```python
from build123d import *

# Parameters (mm, degrees)
ESQUISSE1_R             = 1.6
EXTRUSION1_DEPTH        = 1
ESQUISSE2_W             = 59.55
ESQUISSE2_H             = 1
EXTRUSION2_DEPTH        = 7
ESQUISSE3_W             = 92.55
ESQUISSE3_H             = 1
EXTRUSION3_DEPTH        = 7.5
ESQUISSE4_W             = 92.55
ESQUISSE4_H             = 1
EXTRUSION4_DEPTH        = 8
CONG_1_R                = 1
CONG_2_R                = 2
CONG_3_R                = 1
CONG_4_R                = 2
ESQUISSE5_W             = 1.5
ESQUISSE5_H             = 17
ENL_V_MAT_EXTRU_1_DEPTH = 10
CONG_5_R                = 0.75
CONG_6_R                = 0.74
CONG_7_R                = 0.74
CONG_8_R                = 0.75


with BuildPart() as part:
    # Esquisse1 → Extrusion1 (new body)
    with BuildSketch(Plane.XY):
        Polygon((-46.275, -25.41), (-25.275, -25.41), (-25.275, -39.22), (34.275, -39.22), (34.275, -25.41), (46.275, -25.41), (46.275, -49.22), (-46.275, -49.22), align=None)
        with Locations((37.275, -29.41)):
            Circle(ESQUISSE1_R, mode=Mode.SUBTRACT)
        with Locations((-37.275, -29.41)):
            Circle(ESQUISSE1_R, mode=Mode.SUBTRACT)
    extrude(amount=EXTRUSION1_DEPTH)

    # Esquisse2 → Extrusion2 (add)
    with BuildSketch(Plane.XY.offset(1)):
        with Locations((4.5, -39.72)):
            Rectangle(ESQUISSE2_W, ESQUISSE2_H)
    extrude(amount=-EXTRUSION2_DEPTH)

    # Esquisse3 → Extrusion3 (add)
    with BuildSketch(Plane.XY.offset(1)):
        with Locations((0, -49.72)):
            Rectangle(ESQUISSE3_W, ESQUISSE3_H)
    extrude(amount=-EXTRUSION3_DEPTH)

    # Esquisse4 → Extrusion4 (add)
    with BuildSketch(Plane.XZ.offset(50.22)):
        with Locations((0, -6)):
            Rectangle(ESQUISSE4_W, ESQUISSE4_H)
    extrude(amount=EXTRUSION4_DEPTH)

    # Congé1
    cong_1_edges = [part.edges().sort_by_distance(p)[0] for p in [
        (0, -50.22, -5.5),
        (0, -49.22, 0),
    ]]
    fillet(cong_1_edges, radius=CONG_1_R)

    # Congé2
    cong_2_edges = [part.edges().sort_by_distance(p)[0] for p in [
        (0, -49.22, -6.5),
        (0, -50.22, 1),
    ]]
    fillet(cong_2_edges, radius=CONG_2_R)

    # Congé3
    cong_3_edges = [part.edges().sort_by_distance(p)[0] for p in [
        (4.5, -40.22, 0),
    ]]
    fillet(cong_3_edges, radius=CONG_3_R)

    # Congé4
    # the kernel refuses this fillet: 2 mm, written as the material it takes off along each edge
    with BuildSketch(Plane(origin=(-25.275, -39.22, 1), x_dir=(0, -1, 0), z_dir=(1, 0, 0))) as cong_4_piece_1:
        with BuildLine():
            CenterArc((CONG_4_R, CONG_4_R), CONG_4_R, 180, 90)
            Line((0, CONG_4_R), (0, 0))
            Line((0, 0), (CONG_4_R, 0))
        make_face()
    extrude(amount=59.55, mode=Mode.SUBTRACT)

    # Esquisse5 → Enlèv. mat.-Extru.1 (cut)
    with BuildSketch(Plane.XY.offset(1)):
        with Locations((-24.525, -33.91)):
            Rectangle(ESQUISSE5_W, ESQUISSE5_H)
        with Locations((33.525, -33.91)):
            Rectangle(ESQUISSE5_W, ESQUISSE5_H)
    extrude(amount=-ENL_V_MAT_EXTRU_1_DEPTH, mode=Mode.SUBTRACT)

    # Congé5
    cong_5_edges = [part.edges().sort_by_distance(p)[0] for p in [
        (-25.275, -42.41, 0.5),
    ]]
    fillet(cong_5_edges, radius=CONG_5_R)

    # Congé6
    cong_6_edges = [part.edges().sort_by_distance(p)[0] for p in [
        (-23.775, -42.41, 0.5),
    ]]
    fillet(cong_6_edges, radius=CONG_6_R)

    # Congé7
    cong_7_edges = [part.edges().sort_by_distance(p)[0] for p in [
        (32.775, -42.41, 0.5),
    ]]
    fillet(cong_7_edges, radius=CONG_7_R)

    # Congé8
    cong_8_edges = [part.edges().sort_by_distance(p)[0] for p in [
        (34.275, -42.41, 0.5),
    ]]
    fillet(cong_8_edges, radius=CONG_8_R)


solid = part.part
```
For this review, take the finished solid that the model builds, in its own axes (mm). A direction names the side the tool comes from. Round coordinates to 2 decimals unless told otherwise and drop trailing zeros. Loops run counter-clockwise (first coordinate to the right, second up) from the corner with the lowest first, then second, coordinate; pieces in that order, holes last.
Q1. Add section D-D on y = -47. Write out the cut boundary in (x, z) (3 decimals).
Result sheet:
outline: (-46.275, 0) - (46.275, 0) - (46.275, 1) - (-46.275, 1) - close
Q2. Mouldability with a two-part tool opening along Y and no side actions: class faces 5 (the face through (1, -42, 0)), 6 (the face through (-23.775, -40, -2)), 7 (the face through (4.1, -39.79, 0.4)) as +Y half, -Y half, draft (parallel to the pull), parting line (faces both ways), or undercut.
Result sheet:
face 5: undercut
face 6: draft
face 7: +Y half
Q3. Machinability: for faces 1 (the face through (-1, -55, -5.5)), 2 (the face through (0.65, -49.82, -5.93)), 3 (the face through (-1, -42, 1)), 4 (the face through (32.775, -40, -2)), which of the approach directions +Z, -Z, +X, -X, +Y, -Y give a long, thin tool a straight path to every point of the face, cutting with its end or side? Answer none if there is none.
Result sheet:
face 1: +Z, +X, -X, -Y
face 2: -Z, +X, -X
face 3: +Z, +X, -X, +Y, -Y
face 4: +Z, -Z, +Y
Q4. To check wall thickness, follow line 1 along X through (y, z) = (-35, 0.5) (3 decimals); line 2 along Y through (x, z) = (-16.5, -4.5); line 3 along Z through (x, y) = (-9, -42). State the ranges of each line that lie inside material, in increasing order.
Result sheet:
line 1: x = -46.275 to -25.275, 34.275 to 46.275
line 2: y = -50.22 to -49.22, -40.22 to -39.22
line 3: z = 0 to 1
Q5. Add section B-B on y = -29.41. Write out the cut boundary in (x, z) (3 decimals), plus the area to 3 significant figures.
Result sheet:
outline: (-46.275, 0) - (-38.875, 0) - (-38.875, 1) - (-46.275, 1) - close; (-35.675, 0) - (-25.275, 0) - (-25.275, 1) - (-35.675, 1) - close; (34.275, 0) - (35.675, 0) - (35.675, 1) - (34.275, 1) - close; (38.875, 0) - (46.275, 0) - (46.275, 1) - (38.875, 1) - close
area: 26.6 mm2
Q6. Insertion check: pin 1 Ø7 at (x, y) = (12.5, -38.5) entering from -Z; pin 2 Ø1.5 at (x, z) = (-1.5, -2.5) entering from -Y; pin 3 Ø4 at (x, z) = (25.5, -5) entering from +Y; pin 4 Ø5 at (x, y) = (34, -37) entering from +Z. Each pin has a flat end and moves straight along its axis. Give the tip position at first contact, or say it passes through.
Result sheet:
pin 1: stops at z = -6
pin 2: stops at y = -50.22
pin 3: stops at y = -39.22
pin 4: stops at z = 1
Q7. Add section A-A on y = -34. Write out the cut boundary in (x, z) (3 decimals).
Result sheet:
outline: (-46.275, 0) - (-25.275, 0) - (-25.275, 1) - (-46.275, 1) - close; (34.275, 0) - (46.275, 0) - (46.275, 1) - (34.275, 1) - close
Q8. Add section C-C on x = -3. Write out the cut boundary in (y, z), plus the area to 3 significant figures.
Result sheet:
outline: (-58.22, -6.5) - (-51.22, -6.5) arc R2 ccw to (-49.22, -4.5) - (-49.22, -1) arc R1 cw to (-48.22, 0) - (-41.22, 0) arc R1 cw to (-40.22, -1) - (-40.22, -6) - (-39.22, -6) - (-39.22, -1) arc R2 ccw to (-41.22, 1) - (-48.22, 1) arc R2 ccw to (-50.22, -1) - (-50.22, -4.5) arc R1 cw to (-51.22, -5.5) - (-58.22, -5.5) - close
area: 29.6 mm2
